Part print with two shaded views. Sizes in mm from the minimum x, y, z corner. Round coordinates to 2 decimals unless told otherwise and drop trailing zeros. Write each loop counter-clockwise with the first axis right and the second up, starting at its lowest first coordinate (ties: lowest second). Pieces come first, ordered by that corner, then holes. Notation, with made-up numbers: (32, -10.75) -> (91, -10.75) arc R10 cw to (91, 1.25) -> close; hole circle Ø9 at (75, 39.5). An arc over 180 degrees is marked (long way). Put each result on its own line as item: value. Start each with the question number.
1. Saw through at A-A on x = 134.62. List the corners of the cut face in (y, z).
2. Drill centre lines: line 1 (Z direction, x = 22.86, y = 3.3); line 2 (X direction, y = 2.35, z = 5.08); line 3 (X direction, y = 58, z = 22). Where is each one in solid material? Low to high. Write a range as from..to.
3. Pull direction Z, two halves, no side cores. Call the marked faces 1 and 2: pulls with the +Z half, pulls with the -Z half, needs draft (parallel to the pull), parting line crosses it, or undercut.
4. Saw through at C-C on x = 73.5. List the corners of the cut face in (y, z), and give its area (3 significant figures).
5. Saw through at D-D on z = 5.08. List the corners of the cut face in (x, y), and give its area (3 significant figures).
6. Flat gauge pins, fed straight in: P1, Ø5.5, axis at y = 1.5, z = 34, coming from the +X side; P2, Ø6.5, axis at x = 30.5, z = 5, coming from the +Y side; P3, Ø6, axis at x = 97.5, y = 40.5, coming from the -Z side. Where does each tip first touch, or does it go through?
7. Saw through at B-B on y = 41. List the corners of the cut face in (x, z), and give its area (3 significant figures).
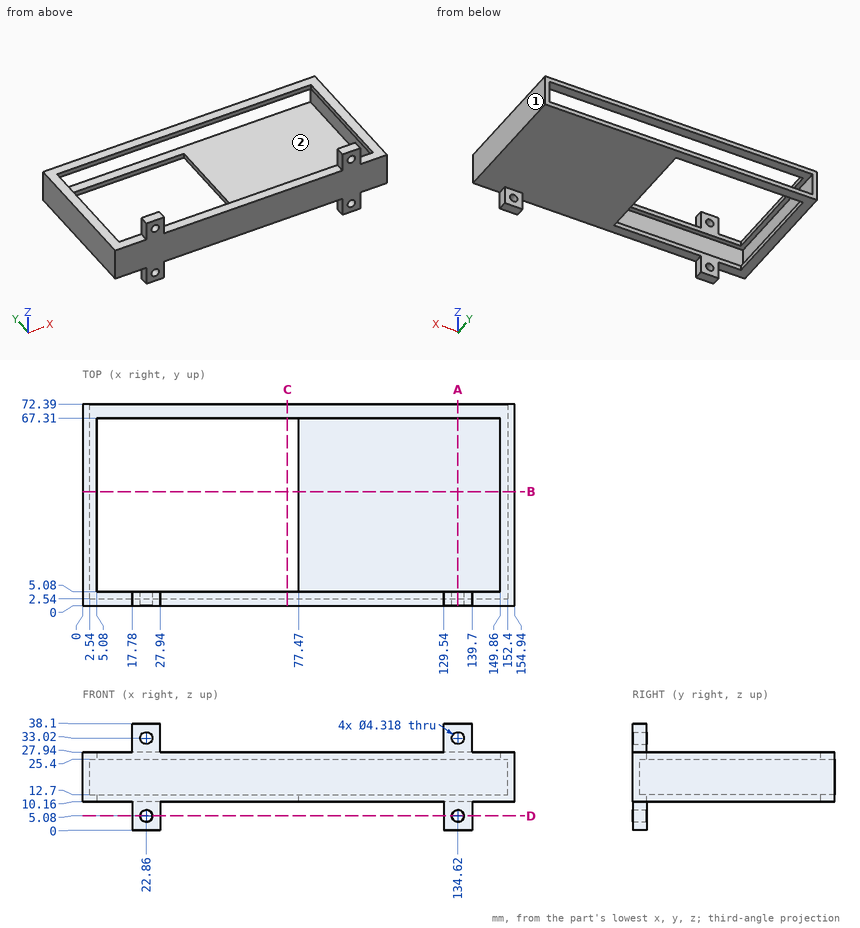
Return value:
1. outline: (0, 0) -> (5.08, 0) -> (5.08, 2.92) -> (0, 2.92) -> close; (0, 7.24) -> (5.08, 7.24) -> (5.08, 10.16) -> (72.39, 10.16) -> (72.39, 12.7) -> (2.54, 12.7) -> (2.54, 25.4) -> (5.08, 25.4) -> (5.08, 30.86) -> (0, 30.86) -> close; (0, 35.18) -> (5.08, 35.18) -> (5.08, 38.1) -> (0, 38.1) -> close; (67.31, 25.4) -> (72.39, 25.4) -> (72.39, 27.94) -> (67.31, 27.94) -> close
2. line 1: z = 0..2.92, 7.24..12.7, 25.4..30.86, 35.18..38.1
2. line 2: x = 17.78..20.7, 25.02..27.94, 129.54..132.46, 136.78..139.7
2. line 3: x = 0..2.54, 152.4..154.94
3. face 1: needs draft
3. face 2: undercut
4. outline: (0, 10.16) -> (5.08, 10.16) -> (5.08, 12.7) -> (2.54, 12.7) -> (2.54, 25.4) -> (5.08, 25.4) -> (5.08, 27.94) -> (0, 27.94) -> close; (67.31, 10.16) -> (72.39, 10.16) -> (72.39, 12.7) -> (67.31, 12.7) -> close; (67.31, 25.4) -> (72.39, 25.4) -> (72.39, 27.94) -> (67.31, 27.94) -> close
4. area: 83.9 mm^2
5. outline: (17.78, 0) -> (20.7, 0) -> (20.7, 5.08) -> (17.78, 5.08) -> close; (25.02, 0) -> (27.94, 0) -> (27.94, 5.08) -> (25.02, 5.08) -> close; (129.54, 0) -> (132.46, 0) -> (132.46, 5.08) -> (129.54, 5.08) -> close; (136.78, 0) -> (139.7, 0) -> (139.7, 5.08) -> (136.78, 5.08) -> close
5. area: 59.4 mm^2
6. P1: stops at x = 139.7
6. P2: stops at y = 5.08
6. P3: stops at z = 10.16
7. outline: (0, 10.16) -> (5.08, 10.16) -> (5.08, 12.7) -> (2.54, 12.7) -> (2.54, 25.4) -> (5.08, 25.4) -> (5.08, 27.94) -> (0, 27.94) -> close; (77.47, 10.16) -> (154.94, 10.16) -> (154.94, 27.94) -> (149.86, 27.94) -> (149.86, 25.4) -> (152.4, 25.4) -> (152.4, 12.7) -> (77.47, 12.7) -> close
7. area: 300 mm^2
